Autodesk Inventor part; units mm, degrees
ref_plane "YZ Plane" through (0, 0, 0) normal (1, 0, 0) x (0, 1, 0)
ref_plane "XZ Plane" through (0, 0, 0) normal (0, 1, 0) x (-1, 0, 0)
ref_plane "XY Plane" through (0, 0, 0) normal (0, 0, 1) x (1, 0, 0)
sketch "Sketch2" plane through (0, 0, 0) normal (0, 0, 1) x (1, 0, 0)
  line L0 (-4, 0) -> (-25, 0)
  line L1 (-25, 0) -> (-25, 17.5)
  line L2 (-25, 17.5) -> (-35, 17.5)
  line L3 (-4, 35) -> (-4, 0)
  line L4 (0, 0) -> (0, 29) construction
  line L5 (-4, 35) -> (-19, 35)
  line L6 (-19, 35) -> (-19, 50)
  line L7 (-35, 17.5) -> (-35, 40.5)
  line L8 (-19, 50) -> (-45, 50)
  line L9 (-45, 50) -> (-45, 40.5)
  line L10 (-45, 40.5) -> (-35, 40.5)
  dimension "d11" = 8
  dimension "d13" = 50
  dimension "d28" = 17.5
  dimension "d29" = 35
  dimension "d30" = 15
  dimension "d34" = 70
  dimension "d35" = 50
  dimension "d36" = 23
  dimension "d37" = 90
revolve "Revolution1" add sketch "Sketch2" angle 360 about axis through (0, 0, 0) along (0, 1, 0)
chamfer "Chamfer1" distance 5 angle 45 1 edges at (19, 50, 0)
properties part number "M17 - Coil Support Part" material "UHMW, Black"
Could you check a few things on this model? Use its own coordinates, in mm. A direction names the side the tool comes from. Coordinates: 2 decimals unless noted, no trailing zeros. Loops run counter-clockwise (first coordinate to the right, second up) from the corner with the lowest first, then second, coordinate; pieces in that order, holes last. Notation, with made-up numbers: (59.25, -24) -> (106.25, -24) arc R29 ccw to (106.25, 9) -> close; hole circle Ø6 at (47, 39.5). An arc over 180 degrees is marked (long way). Answer in a Markdown table with one row per item.
(1) Imagine slicing it at D-D (x = 29.5). List the corners of the cut face in (y, z) for me.
Results found:
| item | result |
|---|---|
| outline | (17.5, -18.83) -> (40.5, -18.83) -> (40.5, -33.98) -> (50, -33.98) -> (50, 33.98) -> (40.5, 33.98) -> (40.5, 18.83) -> (17.5, 18.83) -> close |
(2) Thinking about a two-plate mould opening in Z: for faces 4 (the face through (-19, 50, -19)), 5 (the face through (-8.767, 40.07, -16.856)), 6 (the face through (-17.84, 45.313, -7.397)), 7 (the face through (-23.846, 8.872, 7.509)), which applies, released by +Z, released by -Z, zero draft, split by the parting line, or undercut?
Results found:
| item | result |
|---|---|
| face 4 | zero draft |
| face 5 | undercut |
| face 6 | undercut |
| face 7 | split by the parting line |
(3) Imagine slicing it at A-A (x = 0). List the corners of the cut face in (y, z) for me, plus the area to 4 significant figures.
Results found:
| item | result |
|---|---|
| outline | (0, -25) -> (17.5, -25) -> (17.5, -35) -> (40.5, -35) -> (40.5, -45) -> (50, -45) -> (50, -24) -> (45, -19) -> (35, -19) -> (35, -4) -> (0, -4) -> close; (0, 4) -> (35, 4) -> (35, 19) -> (45, 19) -> (50, 24) -> (50, 45) -> (40.5, 45) -> (40.5, 35) -> (17.5, 35) -> (17.5, 25) -> (0, 25) -> close |
| area | 2,465 mm^2 |
(4) Imagine slicing it at B-B (z = 0). List the corners of the cut face in (x, y) for me.
Results found:
| item | result |
|---|---|
| outline | (-45, 40.5) -> (-35, 40.5) -> (-35, 17.5) -> (-25, 17.5) -> (-25, 0) -> (-4, 0) -> (-4, 35) -> (-19, 35) -> (-19, 45) -> (-24, 50) -> (-45, 50) -> close; (4, 0) -> (25, 0) -> (25, 17.5) -> (35, 17.5) -> (35, 40.5) -> (45, 40.5) -> (45, 50) -> (24, 50) -> (19, 45) -> (19, 35) -> (4, 35) -> close |
(5) Imagine slicing it at C-C (y = 33). List the corners of the cut face in (x, z) for me, plus the area to 3 significant figures.
Results found:
| item | result |
|---|---|
| outline | circle Ø70 at (0, 0); hole circle Ø8 at (0, 0) |
| area | 3,800 mm^2 |
(6) For faces 1 (the face through (0.867, 17.255, 3.905)), 2 (the face through (24, 17.5, 8)), 3 (the face through (0.3, 35, 4.5)), which set-ups out of +Z, -Z, +X, -X, +Y, -Y let a thin tool reach every point of the face, with its end or its side?
Results found:
| item | result |
|---|---|
| face 1 | +Y, -Y |
| face 2 | -Y |
| face 3 | +Y |
(7) Will these pins go through, and if not, where does the flat tip stop? pin 1 Ø6 at (x, z) = (-0.5, 14.5) entering from -Y; pin 2 Ø2 at (y, z) = (10, 22.5) entering from -X; pin 3 Ø23 at (x, z) = (0, 0) entering from +Y; pin 4 Ø12 at (x, y) = (31.5, 44.5) entering from +Z.
Results found:
| item | result |
|---|---|
| pin 1 | stops at y = 0 |
| pin 2 | stops at x = -12.76 |
| pin 3 | stops at y = 35 |
| pin 4 | stops at z = 37.08 |
(8) If I drill on probe 1 along Z at (x, y) = (0, 20.5); probe 2 along X at (y, z) = (29, -2); probe 3 along Y at (x, z) = (2, -34), over which ranges is the centre line in solid material (lowest first)?
Results found:
| item | result |
|---|---|
| probe 1 | z = -35 to -4, 4 to 35 |
| probe 2 | x = -34.94 to -3.46, 3.46 to 34.94 |
| probe 3 | y = 17.5 to 50 |
